Can you work these out from the model? Positions are in its coordinate system, mm. Face numbers are marked on the shaded views. A direction names the side the tool comes from. Coordinates: 2 decimals unless noted, no trailing zeros. Order: outer loops, then holes, each group sorted by start corner. A loop starts at its lowest first (then second) coordinate and runs counter-clockwise, first axis right, second up. Notation, with made-up numbers: M 76,-11 L 128,-11 A15 cw 128,16 Z; hole C -13.75,84.25 d9. An arc over 180 degrees is marked long. Answer as a JSON object with one key per item and string values.
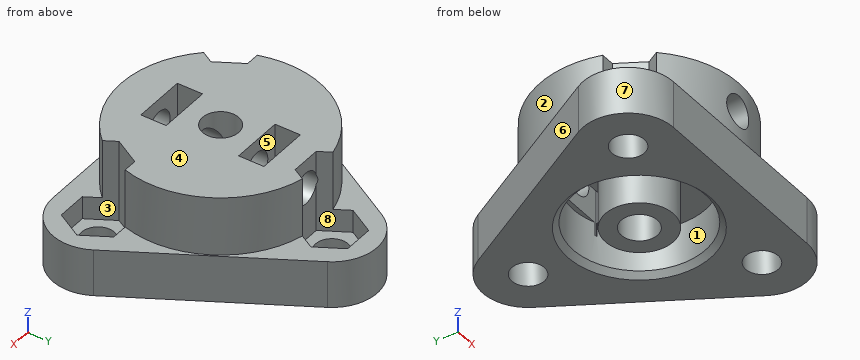
from build123d import *

# Parameters (mm, degrees)
SKETCH_R        = 1.8
PAD_DEPTH       = 5.2
SKETCH002_R     = 11
SKETCH002_R_2   = 2
PAD001_DEPTH    = 6.5
SKETCH003_R     = 7.3
POCKET001_DEPTH = 5.2
POCKET_DEPTH    = 9
SKETCH005_R     = 1.75
POCKET002_DEPTH = 28.451
SKETCH006_W     = 5.8
SKETCH006_H     = 2.8
POCKET003_DEPTH = 8
SKETCH007_R     = 3.75
SKETCH007_R_2   = 2
PAD002_DEPTH    = 5.2
CHAMFER_SIZE    = 0.6


with BuildPart() as part:
    # Sketch → Pad (new body)
    with BuildSketch(Plane.XY):
        with BuildLine():
            Line((-14.982239, -3.65), (-4.330127, 14.8))
            ThreePointArc((4.330127, 14.8), (0, 17.3), (-4.330127, 14.8))
            Line((4.330127, 14.8), (14.982239, -3.65))
            ThreePointArc((10.652112, -11.15), (14.982239, -8.65), (14.982239, -3.65))
            Line((10.652112, -11.15), (-10.652112, -11.15))
            ThreePointArc((-14.982239, -3.65), (-14.982239, -8.65), (-10.652112, -11.15))
        make_face()
        with Locations((0, 12.3)):
            Circle(SKETCH_R, mode=Mode.SUBTRACT)
        with Locations((-10.652112, -6.15)):
            Circle(SKETCH_R, mode=Mode.SUBTRACT)
        with Locations((10.652112, -6.15)):
            Circle(SKETCH_R, mode=Mode.SUBTRACT)
    extrude(amount=PAD_DEPTH)

    # Sketch002 (on Face11 of Pad) → Pad001 (join)
    with BuildSketch(Plane.XY.offset(5.2)):
        Circle(SKETCH002_R)
        Circle(SKETCH002_R_2, mode=Mode.SUBTRACT)
    extrude(amount=PAD001_DEPTH)

    # Sketch003 (on Face4 of Pad001) → Pocket001 (cut)
    with BuildSketch(Plane(origin=(0, 0, 0), x_dir=(1, 0, 0), z_dir=(0, 0, -1))):
        Circle(SKETCH003_R)
    extrude(amount=-POCKET001_DEPTH, mode=Mode.SUBTRACT)

    # Sketch004 (on Face18 of Pocket001) → Pocket (cut)
    with BuildSketch(Plane.XY.offset(11.7)):
        Polygon((-7.303481, -6.15), (-8.977797, -3.25), (-12.326428, -3.25), (-14.000744, -6.15), (-12.326428, -9.05), (-8.977797, -9.05), align=None)
        Polygon((1.674316, 9.4), (3.348632, 12.3), (1.674316, 15.2), (-1.674316, 15.2), (-3.348632, 12.3), (-1.674316, 9.4), align=None)
        Polygon((12.326428, -9.05), (14.000744, -6.15), (12.326428, -3.25), (8.977797, -3.25), (7.303481, -6.15), (8.977797, -9.05), align=None)
    extrude(amount=-POCKET_DEPTH, mode=Mode.SUBTRACT)

    # Sketch005 (on Face6 of Pocket) → Pocket002 (cut, through all)
    with BuildSketch(Plane.XZ.offset(11.15)):
        with Locations((0, 8.5)):
            Circle(SKETCH005_R)
    extrude(amount=-POCKET002_DEPTH, mode=Mode.SUBTRACT)

    # Sketch006 (on Face36 of Pocket002) → Pocket003 (cut)
    with BuildSketch(Plane.XY.offset(11.7)):
        with Locations((0, 5.4)):
            Rectangle(SKETCH006_W, SKETCH006_H)
        with Locations((0, -5.4)):
            Rectangle(SKETCH006_W, SKETCH006_H)
    extrude(amount=-POCKET003_DEPTH, mode=Mode.SUBTRACT)

    # Sketch007 (on Face33 of Pocket003) → Pad002 (join)
    with BuildSketch(Plane(origin=(0, 0, 5.2), x_dir=(1, 0, 0), z_dir=(0, 0, -1))):
        Circle(SKETCH007_R)
        Circle(SKETCH007_R_2, mode=Mode.SUBTRACT)
    extrude(amount=PAD002_DEPTH)

    # Chamfer
    chamfer_edges = [part.edges().sort_by_distance(p)[0] for p in [
        (-7.3, 0, 0),
    ]]
    chamfer(chamfer_edges, length=CHAMFER_SIZE)


solid = part.part
Item 1: I want a section at A-A, the plane y = 0. Write out the boundary of the cut face in (x, z), plus the area to 3 significant figures.
Answers follow:
{"outline": "M -12.87,0 L -7.9,0 L -7.3,0.6 L -7.3,5.2 L -3.75,5.2 L -3.75,0 L -2,0 L -2,11.7 L -11,11.7 L -11,5.2 L -12.87,5.2 Z; M 2,0 L 3.75,0 L 3.75,5.2 L 7.3,5.2 L 7.3,0.6 L 7.9,0 L 12.87,0 L 12.87,5.2 L 11,5.2 L 11,11.7 L 2,11.7 Z", "area": "193 mm^2"}
Item 2: I want a section at C-C, the plane x = 9.5. Write out the boundary of the cut face in (y, z).
Answers follow:
{"outline": "M -11.15,0 L -7.53,0 L -7.53,2.7 L -9.05,2.7 L -9.05,5.2 L -11.15,5.2 Z; M -4.77,0 L 5.85,0 L 5.85,5.2 L 5.55,5.2 L 5.55,11.7 L -3.25,11.7 L -3.25,2.7 L -4.77,2.7 Z"}
Item 3: Which directions (+Z, -Z, +X, -X, +Y, -Y) give clear straight access to the entire face, cutting with the end or side of a thin tool? Please do the marked faces 1, 2, 3, 4 and 5.
Answers follow:
{"face 1": "-Z", "face 2": "+Z, -X", "face 3": "+Z", "face 4": "+Z, +X, -X, +Y, -Y", "face 5": "+Z, -Z"}
Item 4: I want a section at D-D, the plane x = 0. Give the number of separate pieces and of enclosed holes in the cut face, plus the area to 3 significant figures.
Answers follow:
{"separate pieces": "9", "enclosed holes": "0", "area": "98.0 mm^2"}
Item 5: Please list where these lines run through material, in increasing order: line 1 (X direction, y = 0, z = 2.6); line 2 (Z direction, x = 0, y = -9.45); line 3 (Y direction, x = -1.5, z = 2).
Answers follow:
{"line 1": "x = -12.87 to -7.3, -3.75 to -2, 2 to 3.75, 7.3 to 12.87", "line 2": "z = 0 to 6.75, 10.25 to 11.7", "line 3": "y = -11.15 to -7.14, -3.44 to -1.32, 1.32 to 3.44, 7.14 to 11.31, 13.29 to 17.07"}
Item 6: If we mould it in two halves opening along Y, with no side actions, what happens to the marked faces 6, 7 and 8? For each: pulls with the +Y half, pulls with the -Y half, needs draft (parallel to the pull), parting line crosses it, or undercut.
Answers follow:
{"face 6": "pulls with the +Y half", "face 7": "parting line crosses it", "face 8": "undercut"}
Item 7: I'm going to push flat-ended pins straight in: pin 1 (2 mm diameter, centred on y = -5.5, z = 9.5, fed in from +X); pin 2 (0.8 mm diameter, centred on x = 11.5, z = 4, fed in from +Y); pin 3 (6 mm diameter, centred on x = -0.5, z = 9.5, fed in from +Y). Where does each tip first touch, or does it pass through?
Answers follow:
{"pin 1": "stops at x = 8.26", "pin 2": "stops at y = 3.07", "pin 3": "stops at y = 10.73"}
